The listing builds one solid part. Answer for the finished solid, in the listing's coordinates (mm). A direction names the side the tool comes from. Coordinates: 2 decimals unless noted, no trailing zeros. Order: outer loops, then holes, each group sorted by start corner. A loop starts at its lowest first (then second) coordinate and runs counter-clockwise, first axis right, second up. Notation, with made-up numbers: (69, 88) -> (73, 88) arc R13 cw to (73, 113) -> close; hole circle Ø5 at (82, -10.5). An arc over 180 degrees is marked (long way). Write item = value, one per line.
from build123d import *

# Parameters (mm, degrees)
F0_W      = 96
F0_H      = 41
F1_DEPTH  = 24
F2_T      = -1
F3_W      = 69
F3_H      = 19
F4_DEPTH  = 1
F6_W      = 27
F6_H      = 19
F7_DEPTH  = 1
F8_W      = 14
F8_H      = 7
F9_DEPTH  = 2
F10_W     = 3
F10_H     = 4
F11_DEPTH = 1
F12_W     = 5
F12_H     = 6.5
F12_H_2   = 5.5
F13_DEPTH = 18
F14_R     = 1.5
F15_DEPTH = 10
F16_DEPTH = 10


with BuildPart() as f1:
    # F0 (on Top) → F1 (new body)
    with BuildSketch(Plane.XY):
        Rectangle(F0_W, F0_H)
    extrude(amount=F1_DEPTH)

    # F2
    f2_openings = [f1.faces().sort_by_distance(p)[0] for p in [
        (0, 0, 24),
    ]]
    offset(amount=F2_T, openings=f2_openings)

    # F3 (on Front) → F4 (join)
    with BuildSketch(Plane.XZ):
        with Locations((11.5, 9.5)):
            Rectangle(F3_W, F3_H)
    extrude(amount=F4_DEPTH)

    # F6 (on offset) → F7 (join)
    with BuildSketch(Plane.YZ.offset(-24)):
        with Locations((-0.5, 9.5)):
            Rectangle(F6_W, F6_H)
    extrude(amount=F7_DEPTH)

    # F8 (on face) → F9 (cut)
    with BuildSketch(Plane(origin=(-48, 0, 0), x_dir=(0, -1, 0), z_dir=(-1, 0, 0))):
        with Locations((0, 9.5)):
            Rectangle(F8_W, F8_H)
    extrude(amount=-F9_DEPTH, mode=Mode.SUBTRACT)

    # F10 (on face) → F11 (cut)
    with BuildSketch(Plane(origin=(-24, 0, 0), x_dir=(0, -1, 0), z_dir=(-1, 0, 0))):
        with Locations((-3.5, 9)):
            Rectangle(F10_W, F10_H)
        with Locations((3.5, 9)):
            Rectangle(F10_W, F10_H)
    extrude(amount=-F11_DEPTH, mode=Mode.SUBTRACT)

    # F12 (on face) → F13 (join)
    with BuildSketch(Plane.XY.offset(1)):
        with Locations((-25.5, 16.25)):
            Rectangle(F12_W, F12_H)
        with Locations((-25.5, -16.75)):
            Rectangle(F12_W, F12_H_2)
    extrude(amount=F13_DEPTH)

    # F14 (on face) → F15 (cut)
    with BuildSketch(Plane.XY.offset(19)):
        with Locations((-25.5, 16.25)):
            Circle(F14_R)
    extrude(amount=-F15_DEPTH, mode=Mode.SUBTRACT)

    # F14 (on face) → F16 (cut)
    with BuildSketch(Plane.XY.offset(19)):
        with Locations((-25.5, 16.25)):
            Circle(F14_R)
        with Locations((-25.520032, -16.933361)):
            Circle(F14_R)
    extrude(amount=-F16_DEPTH, mode=Mode.SUBTRACT)


solid = f1.part
Q1. Find the intervals of material crossed by line 1 along X through (y, z) = (-13, 11); line 2 along Y through (x, z) = (-11, 6.5); line 3 along X through (y, z) = (-14.5, 2), in increasing order.
The answers:
line_1 = -48 to -47, -24 to -23, 47 to 48
line_2 = -20.5 to -19.5, -1 to 0, 19.5 to 20.5
line_3 = -48 to -47, -28 to -23, 47 to 48
Q2. A tool of negligible diameter and unlimited length cuts with its end or side. For faces 1 (the face through (-1, 0, 0)), 2 (the face through (-23, 10, 10)), from which of +Z, -Z, +X, -X, +Y, -Y can it reach the whole face along a straight path? Write none if from no direction.
The answers:
face_1 = -Z, +X, -X, +Y, -Y
face_2 = +Z
Q3. Each of these flat-tipped pins is pushed along its axis until it touches: pin 1 Ø1.5 at (x, y) = (-6, -14) entering from -Z; pin 2 Ø1 at (y, z) = (3.5, 11) entering from -X; pin 3 Ø10 at (x, y) = (-6.5, 7) entering from +Z. Where does it stop, or does it pass through?
The answers:
pin_1 = 0
pin_2 = -24
pin_3 = 1
Q4. Section B-B, the plane y = 16.25 is taken. Give the vertices of the cut face in (x, z).
The answers:
outline = (-48, 0) -> (48, 0) -> (48, 24) -> (47, 24) -> (47, 1) -> (-23, 1) -> (-23, 19) -> (-24, 19) -> (-24, 9) -> (-27, 9) -> (-27, 19) -> (-28, 19) -> (-28, 1) -> (-47, 1) -> (-47, 24) -> (-48, 24) -> close
Q5. The mould has two halves that part along Y. Classify faces 3 (the face through (-1, 20.5, 12)), 4 (the face through (-24, -1, 10)), 5 (the face through (-48, 0, 14)): released by +Y, released by -Y, zero draft, split by the parting line, or undercut.
The answers:
face_3 = released by +Y
face_4 = undercut
face_5 = zero draft
Q6. Section A-A, the plane x = 31 is taken. Give the vertices of the cut face in (y, z), plus the area to 3 significant figures.
The answers:
outline = (-20.5, 0) -> (20.5, 0) -> (20.5, 24) -> (19.5, 24) -> (19.5, 1) -> (0, 1) -> (0, 19) -> (-1, 19) -> (-1, 1) -> (-19.5, 1) -> (-19.5, 24) -> (-20.5, 24) -> close
area = 105 mm2
Q7. Section C-C, the plane x = -25.5 is taken. Give the vertices of the cut face in (y, z), plus the area to 3 significant figures.
The answers:
outline = (-20.5, 0) -> (20.5, 0) -> (20.5, 24) -> (19.5, 24) -> (19.5, 19) -> (17.75, 19) -> (17.75, 9) -> (14.75, 9) -> (14.75, 19) -> (13, 19) -> (13, 1) -> (-14, 1) -> (-14, 19) -> (-15.43, 19) -> (-15.43, 9) -> (-18.43, 9) -> (-18.43, 19) -> (-19.5, 19) -> (-19.5, 24) -> (-20.5, 24) -> close
area = 243 mm2
